Geometry check sheet. Reference: the model listing, model coordinates, mm. Give positions to 0.01 mm unless a question says otherwise; leave off trailing zeros. Loops run counter-clockwise (first coordinate to the right, second up) from the corner with the lowest first, then second, coordinate; pieces in that order, holes last. Notation, with made-up numbers: (54, -7.75) -> (105, -7.75) arc R11 cw to (105, 10.25) -> close; hole circle Ø9 at (52, -20.5). An arc over 180 degrees is marked (long way). Write each question's results on one line, items separated by ' | '. Start each with the question number.
1) Sectioned sample at A-A on x = 0. Record the cut outline in (y, z).
2) Sectioned sample at B-B on z = 0.6. Record the cut outline in (x, y).
3) Depth check by flat-ended pin: pin 1 (2 mm diameter, centred on x = 0, y = 80, fed in from -Z). Enter the tip coordinate at first touch or a pass-through.
4) Scan lines: line 1 (Y direction, x = 0, z = -0.55); line 2 (X direction, y = 80, z = -0.4); line 3 (Y direction, x = -0.75, z = 1.2). Record each from-to range of solid material in increasing order. Write a range as from..to.
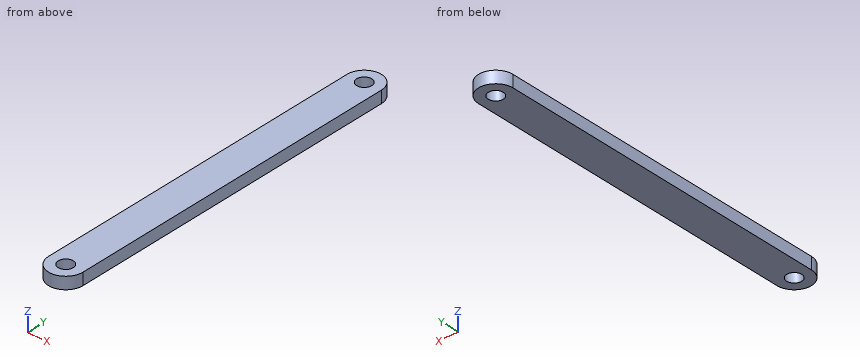
Autodesk Inventor part; units mm, degrees
ref_plane "YZ Plane" through (0, 0, 0) normal (1, 0, 0) x (0, 1, 0)
ref_plane "XZ Plane" through (0, 0, 0) normal (0, 1, 0) x (-1, 0, 0)
ref_plane "XY Plane" through (0, 0, 0) normal (0, 0, 1) x (1, 0, 0)
sketch "Sketch1" plane through (0, 0, 0) normal (0, 0, 1) x (1, 0, 0)
  circle A0 centre (0, 0) radius 4
  line L0 (0, 0) -> (0, 80) construction
  line L1 (4, 0) -> (4, 80)
  line L2 (-4, 80) -> (-4, 0)
  arc A1 (-4, 0) -> (4, 0) centre (0, 0) ccw
  arc A2 (4, 80) -> (-4, 80) centre (0, 80) ccw
  point P0 (0, 40)
  dimension "d0" = 8
  dimension "d1" = 8
  dimension "d2" = 80
extrude "Extrusion1" add sketch "Sketch1" along normal mid plane 2.8
sketch "Sketch2" plane through (0, 0, 1.4) normal (0, 0, 1) x (1, 0, 0)
  arc A0 (4, 80) -> (-4, 80) centre (0, 80) ccw construction
  arc A1 (-4, 0) -> (4, 0) centre (0, 0) ccw construction
  circle A2 centre (0, 0) radius 1.75
  circle A3 centre (0, 80) radius 1.75
  line L0 (0, 12.7) -> (0, 5.7) construction
  line L1 (-1.3, 11.4) -> (-1.3, 7)
  line L2 (1.3, 7) -> (1.3, 11.4)
  arc A4 (1.3, 11.4) -> (-1.3, 11.4) centre (0, 11.4) ccw
  arc A5 (-1.3, 7) -> (1.3, 7) centre (0, 7) ccw
  point P0 (0, 9.2)
  dimension "d5" = 7
  dimension "d6" = 2.6
  dimension "d7" = 7
  dimension "d8" = 3.5
  dimension "d9" = 3.5
extrude "Extrusion2" cut sketch "Sketch2" against normal through all contours A2 | A3
Result:
1) outline: (-4, -1.4) -> (-1.75, -1.4) -> (-1.75, 1.4) -> (-4, 1.4) -> close; (1.75, -1.4) -> (78.25, -1.4) -> (78.25, 1.4) -> (1.75, 1.4) -> close; (81.75, -1.4) -> (84, -1.4) -> (84, 1.4) -> (81.75, 1.4) -> close
2) outline: (-4, 0) arc R4 ccw to (4, 0) -> (4, 80) arc R4 ccw to (-4, 80) -> close; hole circle Ø3.5 at (0, 0); hole circle Ø3.5 at (0, 80)
3) pin 1: through
4) line 1: -4..-1.75, 1.75..78.25, 81.75..84 | line 2: -4..-1.75, 1.75..4 | line 3: -3.93..-1.58, 1.58..78.42, 81.58..83.93
